Input: part model. Units: mm. Frame: model coordinates. Coordinates: 2 decimals unless noted, no trailing zeros. Order: outer loops, then holes, each group sorted by start corner. A loop starts at its lowest first (then second) coordinate and runs counter-clockwise, first axis right, second up. Notation, with made-up numbers: (-14, 14.25) - (19, 14.25) arc R29 cw to (19, 35.25) - close; hole circle Ø10 at (-37.5, 12.5). An arc over 180 degrees is marked (long way). Answer as CSV lines item,"result". Start each with the question number.
Item 1: Section A-A (x = 481). Output: boundary loops of the cut face in (y, z), and give its area (3 significant figures).
Item 2: First-contact query: pin 1 (1.5 mm diameter, centred on x = -260.5, y = -1, fed in from -Z); pin 2 (4 mm diameter, centred on x = 277, z = -75, fed in from +Y). Flat tips, straight axial feed; report the tip coordinate or a pass-through.
Item 3: Material intervals for line 1 along Z through (x, y) = (-326, -2.1); line 2 along Z through (x, y) = (458, -2.3), sorted ascending.
Item 4: Section B-B (z = -10). Output: boundary loops of the cut face in (x, y), and give its area (3 significant figures).
from build123d import *

# Parameters (mm, degrees)
F1_DEPTH    = 2.54
F2_R        = 25.4
F3_T1_DEPTH = 93.0224467373


# Not quite as in the source:
# - a fillet or chamfer that OpenCascade refuses, or shapes differently, is made with other operations: its cross-section is extruded or revolved along the edge and cut away or added


with BuildPart() as f1:
    # F0 (on Front) → F1 (new body)
    with BuildSketch(Plane.XZ):
        Polygon((633.5662589781, 64.4812225811), (-366.4342810219, 64.4812225811), (-366.4342810219, -35.5188314189), (-61.6342810219, -35.5188314189), (255.9216834619, -126.0188282189), (633.5662589781, 4.4813425811), align=None)
    extrude(amount=F1_DEPTH)

    # F2
    f2_edges = [f1.edges().sort_by_distance(p)[0] for p in [
        (633.566259, -1.27, 64.481223),
    ]]
    fillet(f2_edges, radius=F2_R)

    # F3: fillet of radius 25.4 on 1 edges, made by hand

    # F3_s2 → F3_t1 (cut)
    with BuildSketch(Plane.XZ.offset(-45.2412233686)):
        with BuildLine():
            add(Edge.make_bspline(
                [(633.5662589781, 22.5778319285), (633.5662589781, 4.4813425811), (616.4622095682, -1.4291921229)],
                knots=[0, 0, 0, 1, 1, 1], degree=2, weights=[1, 1, 1]))
            Line((616.4622095682, -1.4291921229), (633.5662589781, 4.4813425811))
            Line((633.5662589781, 4.4813425811), (633.5662589781, 22.5778319285))
        make_face()
    extrude(amount=F3_T1_DEPTH, mode=Mode.SUBTRACT)


solid = f1.part
Determined:
1,outline,"(-2.54, -48.24) - (0, -48.24) - (0, 64.48) - (-2.54, 64.48) - close"
1,area,"286 mm^2"
2,pin 1,"stops at z = -35.52"
2,pin 2,"stops at y = 0"
3,line 1,"z = -35.52 to 64.48"
3,line 2,"z = -56.19 to 64.48"
4,outline,"(-366.43, -2.54) - (591.66, -2.54) - (591.66, 0) - (-366.43, 0) - close"
4,area,"2,430 mm^2"
